Print and shaded views of the part. All mm, measured from the part's lowest x, y and z. A direction names the side the tool comes from. Round coordinates to 2 decimals unless told otherwise and drop trailing zeros. Order: outer loops, then holes, each group sorted by start corner. A loop starts at its lowest first (then second) coordinate and runs counter-clockwise, first axis right, second up. Notation, with made-up numbers: M -18.75,45 L 14.25,45 A27 cw 14.25,84 Z; hole C -3.75,45.25 d11. An arc over 180 degrees is marked long. Write each question's results on one line, items separated by ' | '. Start each with the question number.
1. Band-saw the part on C-C, the plane y = 72. List the corners of the cut face in (x, z).
2. Drop flat-ended pins along their axis: pin 1 Ø12 at (y, z) = (46, 21) entering from -X; pin 2 Ø1.5 at (y, z) = (48, 40.5) entering from +X; pin 3 Ø3 at (x, z) = (25, 49.5) entering from +Y; pin 4 Ø10 at (y, z) = (71.5, 18.5) entering from -X. Give the stop position or say it passes through.
3. Band-saw the part on A-A, the plane x = 50. List the corners of the cut face in (y, z).
4. Band-saw the part on B-B, the plane z = 50. List the corners of the cut face in (x, y).
5. Probe L1, parallel to Y at x = 44, z = 50; L2, parallel to X at y = 52.5, z = 27; L3, parallel to Y at x = 14.5, z = 50.5. List the from-to ranges inside material, lowest first. Write a range as [from, to].
6. Which spindle directions (+Z, -Z, +X, -X, +Y, -Y) get a long thin tool onto all of the face, cutting with end or side? Do the marked faces 1, 2 and 3. Say none if no direction does.
7. Band-saw the part on D-D, the plane z = 69.5. List the corners of the cut face in (x, y), then the cut area to 3 significant figures.
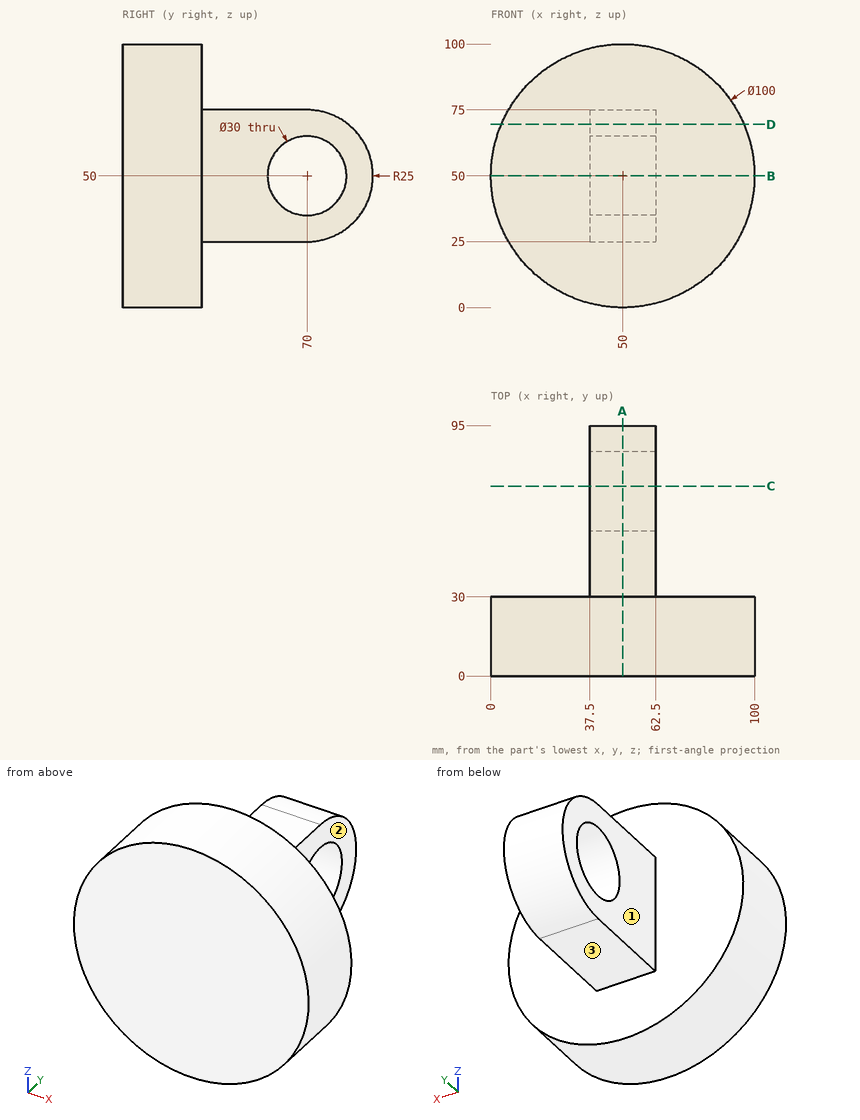
Solution:
1) outline: M 37.5,25.08 L 62.5,25.08 L 62.5,35.13 L 37.5,35.13 Z; M 37.5,64.87 L 62.5,64.87 L 62.5,74.92 L 37.5,74.92 Z
2) pin 1: x = 37.5 | pin 2: x = 62.5 | pin 3: y = 30 | pin 4: through
3) outline: M 0,0 L 30,0 L 30,25 L 70,25 A25 ccw 70,75 L 30,75 L 30,100 L 0,100 Z; hole C 70,50 d30
4) outline: M 0,0 L 100,0 L 100,30 L 62.5,30 L 62.5,55 L 37.5,55 L 37.5,30 L 0,30 Z; M 37.5,85 L 62.5,85 L 62.5,95 L 37.5,95 Z
5) L1: [0, 55], [85, 95] | L2: [37.5, 62.5] | L3: [0, 30]
6) face 1: +Z, -Z, -X, +Y | face 2: +Z, -Z, +X, +Y | face 3: -Z, +X, -X, +Y
7) outline: M 3.96,0 L 96.04,0 L 96.04,30 L 62.5,30 L 62.5,85.64 L 37.5,85.64 L 37.5,30 L 3.96,30 Z | area: 4,150 mm^2
